```python
from build123d import *

# Parameters (mm, degrees)
SKETCH1_W           = 120
SKETCH1_H           = 100
PLATEFORM_DEPTH     = 3
CUT_ARMS_DEPTH      = 10
HOLES_SPACERS_REACH = 158.234
SKETCH6_R           = 1.75


with BuildPart() as part:
    # Sketch1 → plateform (new body)
    with BuildSketch(Plane(origin=(0, 0, 0), x_dir=(1, 0, 0), z_dir=(0, 1, 0))):
        with Locations((60, 50)):
            Rectangle(SKETCH1_W, SKETCH1_H)
    extrude(amount=PLATEFORM_DEPTH)

    # Sketch2 → cut_arms (cut)
    with BuildSketch(Plane(origin=(0, 3, 0), x_dir=(1, 0, 0), z_dir=(0, 1, 0))):
        Polygon((0, 79.562556682), (5, 80), (5, 20), (0, 20.437443318), align=None)
        Polygon((30.437443318, 100), (30, 95), (90, 95), (89.562556682, 100), align=None)
        Polygon((120, 79.562556682), (115, 80), (115, 20), (120, 20.437443318), align=None)
        Polygon((30.437443318, 0), (30, 5), (90, 5), (89.562556682, 0), align=None)
    extrude(amount=-CUT_ARMS_DEPTH, mode=Mode.SUBTRACT)

    # Sketch6 → holes_spacers (cut, up to next)
    with BuildSketch(Plane(origin=(0, 3, 0), x_dir=(1, 0, 0), z_dir=(0, 1, 0)), mode=Mode.PRIVATE) as holes_spacers_sk1:
        with Locations(Location((10.5, 89.5, 0), (0, 0, 270))):
            Circle(SKETCH6_R)
    holes_spacers_tool1 = extrude(holes_spacers_sk1.sketch, amount=-HOLES_SPACERS_REACH, mode=Mode.PRIVATE) & part.part
    # Sketch6 → holes_spacers (cut, up to next)
    with BuildSketch(Plane(origin=(0, 3, 0), x_dir=(1, 0, 0), z_dir=(0, 1, 0)), mode=Mode.PRIVATE) as holes_spacers_sk2:
        with Locations(Location((109.5, 89.5, 0), (0, 0, 270))):
            Circle(SKETCH6_R)
    holes_spacers_tool2 = extrude(holes_spacers_sk2.sketch, amount=-HOLES_SPACERS_REACH, mode=Mode.PRIVATE) & part.part
    # Sketch6 → holes_spacers (cut, up to next)
    with BuildSketch(Plane(origin=(0, 3, 0), x_dir=(1, 0, 0), z_dir=(0, 1, 0)), mode=Mode.PRIVATE) as holes_spacers_sk3:
        with Locations(Location((109.5, 10.5, 0), (0, 0, 270))):
            Circle(SKETCH6_R)
    holes_spacers_tool3 = extrude(holes_spacers_sk3.sketch, amount=-HOLES_SPACERS_REACH, mode=Mode.PRIVATE) & part.part
    # Sketch6 → holes_spacers (cut, up to next)
    with BuildSketch(Plane(origin=(0, 3, 0), x_dir=(1, 0, 0), z_dir=(0, 1, 0)), mode=Mode.PRIVATE) as holes_spacers_sk4:
        with Locations(Location((10.5, 10.5, 0), (0, 0, 270))):
            Circle(SKETCH6_R)
    holes_spacers_tool4 = extrude(holes_spacers_sk4.sketch, amount=-HOLES_SPACERS_REACH, mode=Mode.PRIVATE) & part.part
    add(holes_spacers_tool1.solids().sort_by_distance((10.5, 3, -89.5))[0], mode=Mode.SUBTRACT)
    add(holes_spacers_tool2.solids().sort_by_distance((109.5, 3, -89.5))[0], mode=Mode.SUBTRACT)
    add(holes_spacers_tool3.solids().sort_by_distance((109.5, 3, -10.5))[0], mode=Mode.SUBTRACT)
    add(holes_spacers_tool4.solids().sort_by_distance((10.5, 3, -10.5))[0], mode=Mode.SUBTRACT)


solid = part.part
```
Read the model definition and answer for the solid it produces. Units are mm, in the model's axes. A direction names the side the tool comes from. Give positions to 0.01 mm unless a question says otherwise; leave off trailing zeros. Loops run counter-clockwise (first coordinate to the right, second up) from the corner with the lowest first, then second, coordinate; pieces in that order, holes last.
Item 1: The mould has two halves that part along X. Classify faces 1 (the flat face through (89.784, 1.521, -2.535)), 2 (the flat face through (120, 1, -10)), 3 (the flat face through (59, 0, -51)), 4 (the flat face through (2.535, 1.521, -20.216)): released by +X, released by -X, zero draft, split by the parting line, or undercut.
Item 2: The part is cut by section B-B (y = 1.7). Write down the section's boundary in (x, z).
Item 3: The part is cut by section C-C (z = -10.5). Write down the section's boundary in (x, y).
Item 4: Find the intervals of material crossed by line 1 along Z through (x, y) = (109.5, 1.4); line 2 along X through (y, z) = (1.8, -89.5); line 3 along Z through (x, y) = (59.5, 0.75), in increasing order.
Item 5: The part is cut by section A-A (x = 10.5). Write down the section's boundary in (y, z).
Item 6: The part is cut by section D-D (z = -44.5). Write down the section's boundary in (x, y), and give its area (3 significant figures).
Item 7: For faces 5 (the flat face through (117.535, 1.521, -79.778)), 6 (the flat face through (105, 1, -100)), determine the directions among +Z, -Z, +X, -X, +Y, -Y from which every point of the face is accessible in a straight line to the end or side of a thin tool.
Item 8: Each of these flat-tipped pins is pushed along its axis until it touches: pin 1 Ø1.5 at (y, z) = (1, -35.5) entering from -X; pin 2 Ø5.5 at (x, z) = (109.5, -10.5) entering from -Y; pin 3 Ø1 at (x, y) = (53.5, 2.5) entering from -Z. Where does it stop, or does it pass through?
Taken from the geometry:
1. face 1: undercut
1. face 2: released by +X
1. face 3: zero draft
1. face 4: undercut
2. outline: (0, -100) - (30.44, -100) - (30, -95) - (90, -95) - (89.56, -100) - (120, -100) - (120, -79.56) - (115, -80) - (115, -20) - (120, -20.44) - (120, 0) - (89.56, 0) - (90, -5) - (30, -5) - (30.44, 0) - (0, 0) - (0, -20.44) - (5, -20) - (5, -80) - (0, -79.56) - close; hole circle Ø3.5 at (10.5, -89.5); hole circle Ø3.5 at (10.5, -10.5); hole circle Ø3.5 at (109.5, -89.5); hole circle Ø3.5 at (109.5, -10.5)
3. outline: (0, 0) - (8.75, 0) - (8.75, 3) - (0, 3) - close; (12.25, 0) - (107.75, 0) - (107.75, 3) - (12.25, 3) - close; (111.25, 0) - (120, 0) - (120, 3) - (111.25, 3) - close
4. line 1: z = -100 to -91.25, -87.75 to -12.25, -8.75 to 0
4. line 2: x = 0 to 8.75, 12.25 to 107.75, 111.25 to 120
4. line 3: z = -95 to -5
5. outline: (0, -100) - (3, -100) - (3, -91.25) - (0, -91.25) - close; (0, -87.75) - (3, -87.75) - (3, -12.25) - (0, -12.25) - close; (0, -8.75) - (3, -8.75) - (3, 0) - (0, 0) - close
6. outline: (5, 0) - (115, 0) - (115, 3) - (5, 3) - close
6. area: 330 mm2
7. face 5: +Y, -Y
7. face 6: -Z, +X, -X, +Y, -Y
8. pin 1: stops at x = 5
8. pin 2: stops at y = 0
8. pin 3: stops at z = -95
